Design review of the part built by this model. Coordinates are the model's own, in mm. Face numbers are marked on the shaded views. A direction names the side the tool comes from. Give positions to 0.01 mm unless a question says otherwise; leave off trailing zeros. Loops run counter-clockwise (first coordinate to the right, second up) from the corner with the lowest first, then second, coordinate; pieces in that order, holes last. Notation, with made-up numbers: M 54.5,-7.5 L 100.5,-7.5 A9 cw 100.5,-1.5 Z; hole C 24.25,-16.5 d5. An arc over 180 degrees is marked long. Answer as CSV lines item,"result".
```python
from build123d import *

# Parameters (mm, degrees)
SKETCH1_R           = 1.15
BOSS_EXTRUDE1_DEPTH = 2.9
EXTRUDE_THIN1_DEPTH = 5.8
BOSS_EXTRUDE2_REACH = 15.722
SKETCH4_W           = 0.79
SKETCH4_H           = 0.54
SKETCH5_W           = 0.89
SKETCH5_H           = 2.85
BOSS_EXTRUDE3_DEPTH = 0.56


with BuildPart() as part:
    # Sketch1 → Boss-Extrude1 (new body, symmetric)
    with BuildSketch(Plane.XY):
        Polygon((-6.4, -2.9), (-4.565838245, -2.9), (-4.565838245, -3.592341201), (-1.934161755, -3.592341201), (-1.934161755, -2.9), (1.934161755, -2.9), (1.934161755, -3.592341201), (4.565838245, -3.592341201), (4.565838245, -2.9), (6.4, -2.9), (6.4, 2.9), (-6.4, 2.9), align=None)
        with Locations((-3.25, -2.2)):
            Circle(SKETCH1_R, mode=Mode.SUBTRACT)
        with Locations((3.25, -2.2)):
            Circle(SKETCH1_R, mode=Mode.SUBTRACT)
    extrude(amount=BOSS_EXTRUDE1_DEPTH, both=True)

    # Sketch2 → Extrude-Thin1 (add)
    with BuildSketch(Plane.XY.offset(2.9)):
        Polygon((-5.4, 2.9), (7.557079146, 6.69), (7.58515322, 6.594021636), (-5.371925926, 2.804021636), align=None)
    extrude(amount=-EXTRUDE_THIN1_DEPTH)

    # Sketch4 → Boss-Extrude2 (add, up to next)
    with BuildSketch(Plane(origin=(0, -7.032341201, 0), x_dir=(-1, 0, 0), z_dir=(0, -1, 0)), mode=Mode.PRIVATE) as boss_extrude2_sk1:
        Rectangle(SKETCH4_W, SKETCH4_H)
    boss_extrude2_tool1 = extrude(boss_extrude2_sk1.sketch, amount=-BOSS_EXTRUDE2_REACH, mode=Mode.PRIVATE) - part.part
    add(boss_extrude2_tool1.solids().sort_by_distance((0, -7.032341, 0))[0])
    # Sketch4 → Boss-Extrude2 (add, up to next)
    with BuildSketch(Plane(origin=(0, -7.032341201, 0), x_dir=(-1, 0, 0), z_dir=(0, -1, 0)), mode=Mode.PRIVATE) as boss_extrude2_sk2:
        with Locations((5.1, 0)):
            Rectangle(SKETCH4_W, SKETCH4_H)
    boss_extrude2_tool2 = extrude(boss_extrude2_sk2.sketch, amount=-BOSS_EXTRUDE2_REACH, mode=Mode.PRIVATE) - part.part
    add(boss_extrude2_tool2.solids().sort_by_distance((-5.1, -7.032341, 0))[0])
    # Sketch4 → Boss-Extrude2 (add, up to next)
    with BuildSketch(Plane(origin=(0, -7.032341201, 0), x_dir=(-1, 0, 0), z_dir=(0, -1, 0)), mode=Mode.PRIVATE) as boss_extrude2_sk3:
        with Locations((-5.1, 0)):
            Rectangle(SKETCH4_W, SKETCH4_H)
    boss_extrude2_tool3 = extrude(boss_extrude2_sk3.sketch, amount=-BOSS_EXTRUDE2_REACH, mode=Mode.PRIVATE) - part.part
    add(boss_extrude2_tool3.solids().sort_by_distance((5.1, -7.032341, 0))[0])

    # Sketch5 → Boss-Extrude3 (add)
    with BuildSketch(Plane(origin=(0, 2.9, 0), x_dir=(1, 0, 0), z_dir=(0, 1, 0))):
        with Locations((-2.155, 0)):
            Rectangle(SKETCH5_W, SKETCH5_H)
    extrude(amount=BOSS_EXTRUDE3_DEPTH)


solid = part.part
```
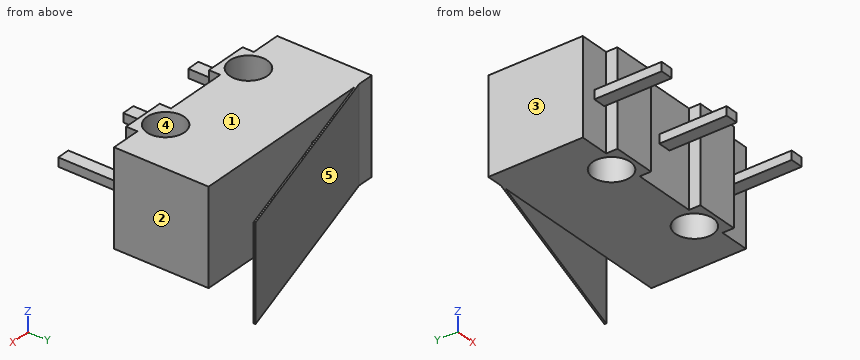
1. We need section C-C, the plane z = 2.25. Write out the cut boundary in (x, y).
Answer block:
outline,"M -6.4,-2.9 L -4.57,-2.9 L -4.57,-3.59 L -1.93,-3.59 L -1.93,-2.9 L 1.93,-2.9 L 1.93,-3.59 L 4.57,-3.59 L 4.57,-2.9 L 6.4,-2.9 L 6.4,2.9 L -5.04,2.9 L 7.59,6.59 L 7.56,6.69 L -5.4,2.9 L -6.4,2.9 Z; hole C -3.25,-2.2 d2.3; hole C 3.25,-2.2 d2.3"
2. For the marked faces 1 and 2, list the 3-axis set-ups (+Z, -Z, +X, -X, +Y, -Y) from which the entire face can be reached by the end or side of a thin tool; tool diameter is ignored.
Answer block:
face 1,"+Z, +X, -X, +Y, -Y"
face 2,"+Z, -Z, +X, -Y"
3. For P1, Ø0.9, axis at x = -5.5, y = -5, coming from the -Z side; P2, Ø1.7, axis at x = 1.5, z = -1, coming from the +Y side; P3, Ø0.9, axis at x = 5.5, y = -5, coming from the +Z side, all flat-tipped, find the tip position at first contact; note any pin that passes through.
Answer block:
P1,"z = -0.27"
P2,"y = 5.17"
P3,"z = 0.27"
4. We need section B-B, the plane x = 2.5. Write out the cut boundary in (y, z).
Answer block:
outline,"M -3.59,-2.9 L -3.07,-2.9 L -3.07,2.9 L -3.59,2.9 Z; M -1.33,-2.9 L 2.9,-2.9 L 2.9,2.9 L -1.33,2.9 Z; M 5.11,-2.9 L 5.21,-2.9 L 5.21,2.9 L 5.11,2.9 Z"
5. We need section A-A, the plane y = -2.2. Write out the cut boundary in (x, z).
Answer block:
outline,"M -6.4,-2.9 L -4.4,-2.9 L -4.4,2.9 L -6.4,2.9 Z; M -2.1,-2.9 L 2.1,-2.9 L 2.1,2.9 L -2.1,2.9 Z; M 4.4,-2.9 L 6.4,-2.9 L 6.4,2.9 L 4.4,2.9 Z"
6. The part is to be moulded in two halves that separate along Y. For the marked faces 3, 4 and 5, say which applies: pulls with the +Y half, pulls with the -Y half, needs draft (parallel to the pull), parting line crosses it, or undercut.
Answer block:
face 3,"needs draft"
face 4,"undercut"
face 5,"pulls with the +Y half"
7. We need section D-D, the plane x = 5. Write out the cut boundary in (y, z), plus the area to 3 significant figures.
Answer block:
outline,"M -7.03,-0.27 L -2.9,-0.27 L -2.9,-2.9 L 2.9,-2.9 L 2.9,2.9 L -2.9,2.9 L -2.9,0.27 L -7.03,0.27 Z; M 5.84,-2.9 L 5.94,-2.9 L 5.94,2.9 L 5.84,2.9 Z"
area,"36.5 mm²"
8. To check wall thickness, follow L1, parallel to X at y = -2.25, z = -2; L2, parallel to X at y = -1.5, z = 0.2; L3, parallel to X at y = 0.5, z = 1.6. State the ranges of each line that lie inside material, in increasing order. Write a range as [from, to].
Answer block:
L1,"[-6.4, -4.4], [-2.1, 2.1], [4.4, 6.4]"
L2,"[-6.4, -4.16], [-2.34, 2.34], [4.16, 6.4]"
L3,"[-6.4, 6.4]"
